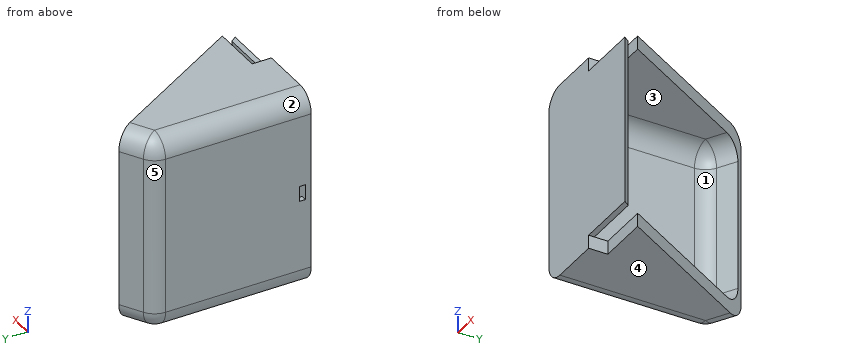
```python
from build123d import *

# Parameters (mm, degrees)
AUFSATZ_LINEAR_AUSTRAGEN1_DEPTH = 7
SKIZZE2_W                       = 35.92542340335845
SKIZZE2_H                       = 3
AUFSATZ_LINEAR_AUSTRAGEN2_DEPTH = 44
SKIZZE4_W                       = 35.92542340335845
SKIZZE4_H                       = 3
AUFSATZ_LINEAR_AUSTRAGEN3_DEPTH = 7
SKIZZE6_W                       = 88
SKIZZE6_H                       = 3
AUFSATZ_LINEAR_AUSTRAGEN4_DEPTH = 32.68
AUFSATZ_LINEAR_AUSTRAGEN5_DEPTH = 88
SKIZZE8_W                       = 8
SKIZZE8_H                       = 3.0000000000000004
SCHNITT_LINEAR_AUSTRAGEN1_DEPTH = 3
VERRUNDUNG1_R                   = 10
VERRUNDUNG2_R                   = 10
SCHNITT_LINEAR_AUSTRAGEN2_DEPTH = 137.3244146724952


with BuildPart() as part:
    # Skizze1 → Aufsatz-Linear austragen1 (new body)
    with BuildSketch(Plane.XY):
        Polygon((-35.925423403358465, 81.63419686002398), (-19.820381056767047, 90.93244739413896), (26.90598923241485, 10.000000000000005), (0, 10.000000000000002), (0, 0), (-35.92542340335845, -4.4e-15), align=None)
    extrude(amount=AUFSATZ_LINEAR_AUSTRAGEN1_DEPTH)

    # Skizze2 → Aufsatz-Linear austragen2 (add)
    with BuildSketch(Plane(origin=(0, 0, 0), x_dir=(-1, 0, 0), z_dir=(0, 0, -1))):
        with Locations((17.962711701679225, 1.5)):
            Rectangle(SKIZZE2_W, SKIZZE2_H)
    aufsatz_linear_austragen2 = extrude(amount=AUFSATZ_LINEAR_AUSTRAGEN2_DEPTH)

    # Spiegeln3: Aufsatz-Linear austragen2 across plane
    add(aufsatz_linear_austragen2.mirror(Plane(origin=(0, 0, -44), x_dir=(1, 0, 0), z_dir=(0, 0, -1))))

    # Skizze4 → Aufsatz-Linear austragen3 (add)
    with BuildSketch(Plane(origin=(0, 0, -88), x_dir=(-1, 0, 0), z_dir=(0, 0, -1))):
        Polygon((-26.905989232414854, 10.000000000000005), (0, 10.000000000000002), (0, 3), (35.92542340335845, 3), (35.925423403358465, 81.63419686002398), (19.820381056767047, 90.93244739413895), align=None)
        with Locations((17.962711701679225, 1.5)):
            Rectangle(SKIZZE4_W, SKIZZE4_H)
    extrude(amount=AUFSATZ_LINEAR_AUSTRAGEN3_DEPTH)

    # Skizze6 → Aufsatz-Linear austragen4 (add)
    with BuildSketch(Plane(origin=(0, 0, 0), x_dir=(0, 0, -1), z_dir=(1, 0, 0))):
        with Locations((44, 1.5)):
            Rectangle(SKIZZE6_W, SKIZZE6_H)
    extrude(amount=AUFSATZ_LINEAR_AUSTRAGEN4_DEPTH)

    # Skizze7 → Aufsatz-Linear austragen5 (add)
    with BuildSketch(Plane.XY.offset(-88)):
        Polygon((-35.92542340335845, 3), (-32.92542340335845, 3), (-32.92542340335845, 79.9021460524551), (-35.925423403358465, 78.17009524488621), align=None)
        Polygon((-35.925423403358465, 78.17009524488621), (-32.92542340335845, 79.9021460524551), (-32.92542340335845, 83.36624766759286), (-35.925423403358465, 81.63419686002398), align=None)
        Polygon((-32.92542340335845, 83.36624766759286), (-32.92542340335845, 79.9021460524551), (-18.32038105676701, 88.33437118278556), (-19.82038105676704, 90.93244739413895), align=None)
    extrude(amount=AUFSATZ_LINEAR_AUSTRAGEN5_DEPTH)

    # Skizze8 → Schnitt-Linear austragen1 (cut)
    with BuildSketch(Plane.ZY.offset(35.92542340335845)):
        with Locations((-43.99999999999999, 4.500000000000002)):
            Rectangle(SKIZZE8_W, SKIZZE8_H)
    extrude(amount=-SCHNITT_LINEAR_AUSTRAGEN1_DEPTH, mode=Mode.SUBTRACT)

    # Verrundung1
    verrundung1_edges = [part.edges().sort_by_distance(p)[0] for p in [
        (-35.92542340335846, 40.81709843001198, 7),
        (-35.925423403358465, 81.63419686002398, -44),
        (-27.872902230062756, 86.28332212708148, 7),
        (-35.92542340335846, 40.81709843001199, -95),
        (-27.872902230062756, 86.28332212708146, -95),
    ]]
    fillet(verrundung1_edges, radius=VERRUNDUNG1_R)

    # Verrundung2
    verrundung2_edges = [part.edges().sort_by_distance(p)[0] for p in [
        (-32.92542340335845, 41.45107302622755, -88),
        (-32.92542340335845, 79.9021460524551, -44),
        (-25.622902230062728, 84.11825861762033, -88),
        (-32.92542340335845, 41.45107302622755, 0),
        (-25.622902230062728, 84.11825861762033, 0),
    ]]
    fillet(verrundung2_edges, radius=VERRUNDUNG2_R)

    # Skizze9 → Schnitt-Linear austragen2 (cut, through all)
    with BuildSketch(Plane.XY):
        Polygon((32.68, 0), (30.488543123002803, 3), (32.68, 3), align=None)
    extrude(amount=-SCHNITT_LINEAR_AUSTRAGEN2_DEPTH, mode=Mode.SUBTRACT)


solid = part.part
```
Here's how the part is built. I have some questions about the finished solid (model axes, mm). Face numbers are marked on the shaded views. A direction names the side the tool comes from. Coordinates: 2 decimals unless noted, no trailing zeros. Loops run counter-clockwise (first coordinate to the right, second up) from the corner with the lowest first, then second, coordinate; pieces in that order, holes last. Notation, with made-up numbers: (89, 56.25) - (101, 56.25) arc R25 cw to (101, 69.25) - close; hole circle Ø2 at (56.25, 6.5). An arc over 180 degrees is marked (long way). Return JSON: item names as keys, results as strings. Group by question number.
Item 1: On a 3-axis mill with a long thin cutter (end or side, diameter ignored), from which of +Z, -Z, +X, -X, +Y, -Y can I reach the whole of each face in a straight line? I mean the marked faces 1 and 2. Say none if no direction works.
Item 2: If we section it at D-D on x = -2.5: Write out the boundary of the cut face in (y, z).
Item 3: We'd pull the mould along Y, two halves only. Please class the marked faces 3, 4 and 5: +Y half, -Y half, draft (parallel to the pull), parting line (faces both ways), or undercut.
Item 4: I need wall thicknesses on line 1 (Z direction, x = -14, y = 13.5); line 2 (Y direction, x = 0, z = -80.5); line 3 (X direction, y = 67, z = -65). Which ranges of each line are inside material? Lowest first, please. Write a range as from..to.
Item 5: Will these pins go through, and if not, where does the flat tip stop? P1, Ø1.5, axis at x = -34.5, y = 5, coming from the +Z side; P2, Ø1, axis at y = 50.5, z = -59, coming from the +X side; P3, Ø3.5, axis at x = 8.5, y = 2, coming from the +Z side.
Item 6: If we section it at A-A on x = 19.5: Write out the boundary of the cut face in (y, z), and give its area (3 significant figures).
Item 7: If we section it at B-B on z = -23: Write out the boundary of the cut face in (x, y).
Item 8: If we section it at C-C on y = 12.5: Write out the boundary of the cut face in (x, z).
Calculated:
{
 "1": {"face 1": "+X", "face 2": "+Z, -X, +Y, -Y"},
 "2": {"outline": "(0, -95) - (60.93, -95) - (60.93, -88) - (3, -88) - (3, 0) - (60.93, 0) - (60.93, 7) - (0, 7) - close"},
 "3": {"face 3": "undercut", "face 4": "draft", "face 5": "+Y half"},
 "4": {"line 1": "z = -95..-88, 0..7", "line 2": "y = 0..3", "line 3": "x = -35.93..-32.93"},
 "5": {"P1": "stops at z = 3.23", "P2": "stops at x = -32.93", "P3": "stops at z = 0"},
 "6": {"outline": "(0, -88) - (3, -88) - (3, 0) - (0, 0) - close; (10, -95) - (22.83, -95) - (22.83, -88) - (10, -88) - close; (10, 0) - (22.83, 0) - (22.83, 7) - (10, 7) - close", "area": "444 mm^2"},
 "7": {"outline": "(-35.93, 0) - (32.68, 0) - (30.49, 3) - (-32.93, 3) - (-32.93, 74.13) arc R10 cw to (-27.93, 82.79) - (-18.32, 88.33) - (-19.82, 90.93) - (-30.93, 84.52) arc R10 ccw to (-35.93, 75.86) - close"},
 "8": {"outline": "(-35.93, -85) arc R10 ccw to (-25.93, -95) - (25.46, -95) - (25.46, -88) - (-22.93, -88) arc R10 cw to (-32.93, -78) - (-32.93, -10) arc R10 cw to (-22.93, 0) - (25.46, 0) - (25.46, 7) - (-25.93, 7) arc R10 ccw to (-35.93, -3) - close"}
}
